Verification items for the finished model (mm, model axes). Face numbers are marked on the shaded views. A direction names the side the tool comes from. Round coordinates to 2 decimals unless told otherwise and drop trailing zeros. Loops run counter-clockwise (first coordinate to the right, second up) from the corner with the lowest first, then second, coordinate; pieces in that order, holes last. Notation, with made-up numbers: (87.25, -31) - (136.25, -31) arc R22 cw to (136.25, 2) - close; hole circle Ø2 at (59, 31.5). An arc over 180 degrees is marked (long way). Use a Markdown table: item, result. Add a question column.
```python
from build123d import *

# Parameters (mm, degrees)
SKETCH1_R             = 1.5
BOSS_EXTRUDE1_DEPTH   = 2
BOSS_EXTRUDE1_2_DEPTH = 2
BOSS_EXTRUDE1_3_DEPTH = 2
BOSS_EXTRUDE1_4_DEPTH = 2
SKETCH1_3_W           = 20
SKETCH1_3_H           = 5
BOSS_EXTRUDE2_DEPTH   = 1
SKETCH1_4_R           = 0.75
CUT_EXTRUDE1_DEPTH    = 1
SKETCH1_6_W           = 20
SKETCH1_6_H           = 5
SKETCH1_6_W_2         = 18
SKETCH1_6_H_2         = 3
SKETCH1_6_R           = 1
BOSS_EXTRUDE4_DEPTH   = 5


with BuildPart() as part:
    # Sketch1 → Boss-Extrude1 (new body)
    with BuildSketch(Plane(origin=(0, 0, 0), x_dir=(1, 0, 0), z_dir=(0, 1, 0))):
        with Locations(Location((-7.5, 0, 0), (0, 0, 270))):
            Circle(SKETCH1_R)
    extrude(amount=BOSS_EXTRUDE1_DEPTH)



with BuildPart() as body_2:
    # Sketch1 → Boss-Extrude1 2 (new body)
    with BuildSketch(Plane(origin=(0, 0, 0), x_dir=(1, 0, 0), z_dir=(0, 1, 0))):
        with Locations(Location((-2.5, 0, 0), (0, 0, 270))):
            Circle(SKETCH1_R)
    extrude(amount=BOSS_EXTRUDE1_2_DEPTH)


with BuildPart() as body_3:
    # Sketch1 → Boss-Extrude1 3 (new body)
    with BuildSketch(Plane(origin=(0, 0, 0), x_dir=(1, 0, 0), z_dir=(0, 1, 0))):
        with Locations(Location((2.5, 0, 0), (0, 0, 270))):
            Circle(SKETCH1_R)
    extrude(amount=BOSS_EXTRUDE1_3_DEPTH)


with BuildPart() as body_4:
    # Sketch1 → Boss-Extrude1 4 (new body)
    with BuildSketch(Plane(origin=(0, 0, 0), x_dir=(1, 0, 0), z_dir=(0, 1, 0))):
        with Locations(Location((7.5, 0, 0), (0, 0, 270))):
            Circle(SKETCH1_R)
    extrude(amount=BOSS_EXTRUDE1_4_DEPTH)


with BuildPart() as part_1:
    add(part.part)

    add(body_2.part)  # Boss-Extrude2 merges body 2

    add(body_3.part)  # Boss-Extrude2 merges body 3

    add(body_4.part)  # Boss-Extrude2 merges body 4
    # Sketch1_3 → Boss-Extrude2 (add)
    with BuildSketch(Plane(origin=(0, 0, 0), x_dir=(1, 0, 0), z_dir=(0, 1, 0))):
        Rectangle(SKETCH1_3_W, SKETCH1_3_H)
    extrude(amount=BOSS_EXTRUDE2_DEPTH)

    # Sketch1_4 → Cut-Extrude1 (cut)
    with BuildSketch(Plane(origin=(0, 0, 0), x_dir=(1, 0, 0), z_dir=(0, 1, 0))):
        with Locations(Location((-7.5, 0, 0), (0, 0, 270))):
            Circle(SKETCH1_4_R)
        with Locations(Location((-2.5, 0, 0), (0, 0, 270))):
            Circle(SKETCH1_4_R)
        with Locations(Location((2.5, 0, 0), (0, 0, 270))):
            Circle(SKETCH1_4_R)
        with Locations(Location((7.5, 0, 0), (0, 0, 270))):
            Circle(SKETCH1_4_R)
    extrude(amount=CUT_EXTRUDE1_DEPTH, mode=Mode.SUBTRACT)

    # Sketch1_6 → Boss-Extrude4 (add)
    with BuildSketch(Plane(origin=(0, 0, 0), x_dir=(1, 0, 0), z_dir=(0, 1, 0))):
        Rectangle(SKETCH1_6_W, SKETCH1_6_H)
        Rectangle(SKETCH1_6_W_2, SKETCH1_6_H_2, mode=Mode.SUBTRACT)
        with BuildLine():
            ThreePointArc((-4, 0), (-5, 1), (-6, 0))
            Line((-6, 0), (-4, 0))
        make_face()
        with BuildLine():
            Line((-4, 0), (-6, 0))
            ThreePointArc((-6, 0), (-5, -1), (-4, 0))
        make_face()
        with Locations(Location((0, 0, 0), (0, 0, 270))):
            Circle(SKETCH1_6_R)
        with Locations(Location((5, 0, 0), (0, 0, 270))):
            Circle(SKETCH1_6_R)
    extrude(amount=-BOSS_EXTRUDE4_DEPTH)


solid = part_1.part
```
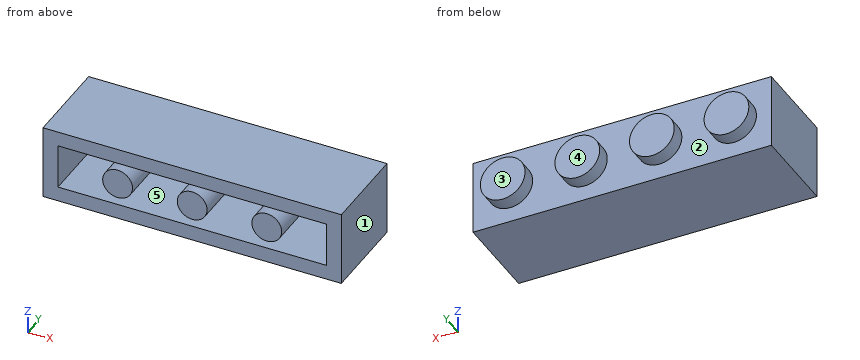
Q1. Thickness scan on line 1 along X through (y, z) = (0.45, 0); line 2 along X through (y, z) = (-1.25, -0.1); line 3 along Z through (x, y) = (7, -2). Record the ranges inside material, lowest first.
Q2. Section check D-D on x = -5. Record the cut outline in (y, z), plus the area to 3 significant figures.
Q3. Section check A-A on y = -3.25. Record the cut outline in (x, z).
Q4. Section check B-B on x = 7.5. Record the cut outline in (y, z).
Q5. Release check for a two-part mould opening along X. For the marked faces 1, 2 and 3 record: +X half, -X half, draft (parallel to the pull), parting line (faces both ways), or undercut.
Q6. Set-up check for the marked faces 4 and 5: record each of +Z, -Z, +X, -X, +Y, -Y from which the full face is reachable in a straight line by a thin tool's end or side.
Q7. Section check C-C on y = 1.5. Record the cut outline in (x, z), plus the area to 3 significant figures.
Q8. Go/stop test with flat-tipped pins: pin 1 Ø1.4 at (x, z) = (-7.5, 0) entering from -Y; pin 2 Ø0.8 at (x, z) = (8, 0) entering from -Y. Record where each tip stops, or that it passes through.
Determined:
| question | item | result |
|---|---|---|
| 1 | line 1 | x = -10 to -8.25, -6.75 to -3.25, -1.75 to 1.75, 3.25 to 6.75, 8.25 to 10 |
| 1 | line 2 | x = -10 to -9, -5.99 to -4.01, -0.99 to 0.99, 4.01 to 5.99, 9 to 10 |
| 1 | line 3 | z = -2.5 to -1.5, 1.5 to 2.5 |
| 2 | outline | (-5, -2.5) - (1, -2.5) - (1, 2.5) - (-5, 2.5) - (-5, 1.5) - (0, 1.5) - (0, 1) - (-5, 1) - (-5, -1) - (0, -1) - (0, -1.5) - (-5, -1.5) - close |
| 2 | area | 25.0 mm² |
| 3 | outline | (-10, -2.5) - (10, -2.5) - (10, 2.5) - (-10, 2.5) - close; circle Ø2 at (-5, 0); circle Ø2 at (0, 0); circle Ø2 at (5, 0); hole (-9, -1.5) - (9, -1.5) - (9, 1.5) - (-9, 1.5) - close |
| 4 | outline | (-5, -2.5) - (1, -2.5) - (1, -1.5) - (2, -1.5) - (2, 1.5) - (1, 1.5) - (1, 2.5) - (-5, 2.5) - (-5, 1.5) - (0, 1.5) - (0, 0.75) - (1, 0.75) - (1, -0.75) - (0, -0.75) - (0, -1.5) - (-5, -1.5) - close |
| 5 | face 1 | +X half |
| 5 | face 2 | undercut |
| 5 | face 3 | draft |
| 6 | face 4 | +Z, -Z, +X, -X, +Y |
| 6 | face 5 | -Y |
| 7 | outline | circle Ø3 at (-7.5, 0); circle Ø3 at (-2.5, 0); circle Ø3 at (2.5, 0); circle Ø3 at (7.5, 0) |
| 7 | area | 28.3 mm² |
| 8 | pin 1 | stops at y = 1 |
| 8 | pin 2 | stops at y = 0 |
